Can you work these out from the model? Positions are in its coordinate system, mm. A direction names the side the tool comes from. Coordinates: 2 decimals unless noted, no trailing zeros. Loops run counter-clockwise (first coordinate to the right, second up) from the corner with the lowest first, then second, coordinate; pieces in that order, holes last.
```python
from build123d import *

# Parameters (mm, degrees)
SKETCH1_W           = 13
SKETCH1_H           = 17
BOSS_EXTRUDE1_DEPTH = 2
BOSS_EXTRUDE2_DEPTH = 10
SKETCH3_R           = 5.75
CUT_EXTRUDE1_DEPTH  = 15
SKETCH4_W           = 17
SKETCH4_H           = 37
BOSS_EXTRUDE3_DEPTH = 2
SKETCH5_W           = 17
SKETCH5_H           = 2
BOSS_EXTRUDE4_DEPTH = 4.5
BOSS_EXTRUDE5_DEPTH = 0.9
SKETCH7_W           = 0.5
SKETCH7_H           = 24.1
BOSS_EXTRUDE6_DEPTH = 0.9
SKETCH8_W           = 7.4
SKETCH8_H           = 0.5
BOSS_EXTRUDE7_DEPTH = 0.9
BOSS_EXTRUDE8_DEPTH = 17


with BuildPart() as part:
    # Sketch1 → Boss-Extrude1 (new body)
    with BuildSketch(Plane(origin=(0, 0, 0), x_dir=(1, 0, 0), z_dir=(0, 1, 0))):
        Rectangle(SKETCH1_W, SKETCH1_H)
    extrude(amount=BOSS_EXTRUDE1_DEPTH)

    # Sketch2 → Boss-Extrude2 (add)
    with BuildSketch(Plane(origin=(0, 2, 0), x_dir=(1, 0, 0), z_dir=(0, 1, 0))):
        Polygon((-6.5, 8.5), (-6.5, -8.5), (6.5, -8.5), (6.5, -6.5), (-4.5, -6.5), (-4.5, 6.5), (6.5, 6.5), (6.5, 8.5), align=None)
    extrude(amount=BOSS_EXTRUDE2_DEPTH)

    # Sketch3 → Cut-Extrude1 (cut)
    with BuildSketch(Plane.ZY.offset(6.5)):
        with Locations((0, 10)):
            Circle(SKETCH3_R)
    extrude(amount=-CUT_EXTRUDE1_DEPTH, mode=Mode.SUBTRACT)

    # Sketch4 → Boss-Extrude3 (add)
    with BuildSketch(Plane(origin=(6.5, 0, 0), x_dir=(0, 0, -1), z_dir=(1, 0, 0))):
        with Locations((0, 18.5)):
            Rectangle(SKETCH4_W, SKETCH4_H)
    extrude(amount=BOSS_EXTRUDE3_DEPTH)

    # Sketch5 → Boss-Extrude4 (add)
    with BuildSketch(Plane(origin=(8.5, 0, 0), x_dir=(0, 0, -1), z_dir=(1, 0, 0))):
        with Locations((0, 36)):
            Rectangle(SKETCH5_W, SKETCH5_H)
    extrude(amount=BOSS_EXTRUDE4_DEPTH)

    # Sketch6 → Boss-Extrude5 (add)
    with BuildSketch(Plane(origin=(0, 12, 0), x_dir=(1, 0, 0), z_dir=(0, 1, 0))):
        Polygon((-6, 5.390964663), (-6.5, 5.390964663), (-6.5, 8.5), (6.5, 8.5), (6.5, 8), (-6, 8), align=None)
        Polygon((6.5, -8), (-6, -8), (-6, -5.390964663), (-6.5, -5.390964663), (-6.5, -8.5), (6.5, -8.5), align=None)
    extrude(amount=BOSS_EXTRUDE5_DEPTH)

    # Sketch7 → Boss-Extrude6 (add)
    with BuildSketch(Plane.ZY.offset(-6.5)):
        with Locations((-8.25, 24.95)):
            Rectangle(SKETCH7_W, SKETCH7_H)
        with Locations((8.25, 24.95)):
            Rectangle(SKETCH7_W, SKETCH7_H)
    extrude(amount=BOSS_EXTRUDE6_DEPTH)

    # Sketch8 → Boss-Extrude7 (add)
    with BuildSketch(Plane(origin=(0, 37, 0), x_dir=(1, 0, 0), z_dir=(0, 1, 0))):
        with Locations((9.3, 8.25)):
            Rectangle(SKETCH8_W, SKETCH8_H)
        with Locations((9.3, -8.25)):
            Rectangle(SKETCH8_W, SKETCH8_H)
    extrude(amount=BOSS_EXTRUDE7_DEPTH)

    # Sketch9 → Boss-Extrude8 (add)
    with BuildSketch(Plane.XY.offset(8.5)):
        Polygon((13, 35), (8.5, 30.5), (8.5, 35), align=None)
    extrude(amount=-BOSS_EXTRUDE8_DEPTH)


solid = part.part
```
(1) I want a section at D-D on x = 9.75. Write out the boundary of the cut face in (y, z).
Check values:
outline: (31.75, -8.5) - (37.9, -8.5) - (37.9, -8) - (37, -8) - (37, 8) - (37.9, 8) - (37.9, 8.5) - (31.75, 8.5) - close
(2) I want a section at C-C on y = 12.5. Write out the boundary of the cut face in (x, z).
Check values:
outline: (-6.5, -8.5) - (8.5, -8.5) - (8.5, 8.5) - (-6.5, 8.5) - (-6.5, 5.39) - (-6, 5.39) - (-6, 8) - (6.5, 8) - (6.5, -8) - (-6, -8) - (-6, -5.39) - (-6.5, -5.39) - close
(3) If we mould it in two halves opening along Z, with no side actions, what happens to faces 1 (the flat face through (3, 12, 8.5)), 2 (the flat face through (13, 36, 0)), 3 (the flat face through (-6, 12.4, 6.7))? For each: released by +Z, released by -Z, zero draft, split by the parting line, or undercut.
Check values:
face 1: released by +Z
face 2: zero draft
face 3: undercut
(4) I want a section at A-A on z = 0. Write out the boundary of the cut face in (x, y).
Check values:
outline: (-6.5, 0) - (8.5, 0) - (8.5, 30.5) - (13, 35) - (13, 37) - (6.5, 37) - (6.5, 2) - (-4.5, 2) - (-4.5, 4.25) - (-6.5, 4.25) - close
(5) I want a section at B-B on x = 5. Write out the boundary of the cut face in (y, z), then the cut area to 3 significant figures.
Check values:
outline: (0, -8.5) - (12.9, -8.5) - (12.9, -8) - (12, -8) - (12, -6.5) - (2, -6.5) - (2, 6.5) - (12, 6.5) - (12, 8) - (12.9, 8) - (12.9, 8.5) - (0, 8.5) - close
area: 74.9 mm2
(6) Which directions (+Z, -Z, +X, -X, +Y, -Y) give clear straight access to the entire face, cutting with the end or side of a thin tool? Please do faces 4 (the flat face through (-1.8, 12.9, 8.2)), 5 (the flat face through (10, 37, 0)), 6 (the flat face through (6, 23, -8)).
Check values:
face 4: +Z, -Z, -X, +Y
face 5: +X, -X, +Y
face 6: +Y
(7) I'm going to push flat-ended pins straight in: pin 1 (3 mm diameter, centred on x = 9, z = 2, fed in from +Y); pin 2 (1.3 mm diameter, centred on x = 1.5, z = -6.5, fed in from +Y); pin 3 (1.5 mm diameter, centred on x = 9.5, z = 6.5, fed in from -Y). Where does each tip first touch, or does it pass through?
Check values:
pin 1: stops at y = 37
pin 2: stops at y = 12
pin 3: stops at y = 30.75
(8) If I drill on probe 1 along Z at (x, y) = (-3, 6); probe 2 along Z at (x, y) = (-5.85, 10); probe 3 along Y at (x, z) = (-5.2, 0), over which ranges is the centre line in solid material (lowest first)?
Check values:
probe 1: z = -8.5 to -6.5, 6.5 to 8.5
probe 2: z = -8.5 to -5.75, 5.75 to 8.5
probe 3: y = 0 to 4.25
